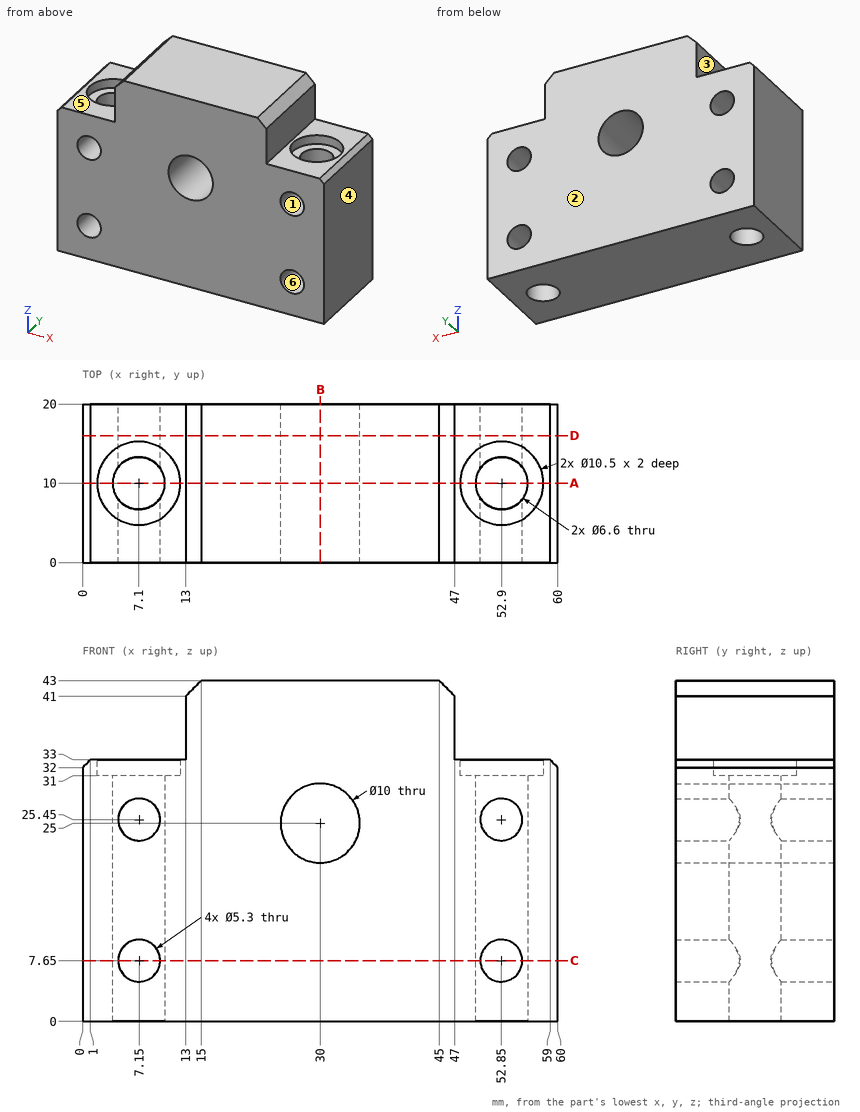
Drawing for the job (mm, zero at the part's lowest x, y, z). A direction names the side the tool comes from. Coordinates: 2 decimals unless noted, no trailing zeros. Order: outer loops, then holes, each group sorted by start corner. A loop starts at its lowest first (then second) coordinate and runs counter-clockwise, first axis right, second up.
Item 1: Band-saw the part on C-C on z = 7.65. List the corners of the cut face in (x, y), plus the area to 3 significant figures.
Check sheet entries:
outline: (0, 0) - (4.5, 0) - (4.5, 7.97) arc R3.3 cw to (4.5, 12.03) - (4.5, 20) - (0, 20) - close; (9.8, 0) - (50.2, 0) - (50.2, 8.1) arc R3.3 cw to (50.2, 11.9) - (50.2, 20) - (9.8, 20) - (9.8, 11.9) arc R3.3 cw to (9.8, 8.1) - close; (55.5, 0) - (60, 0) - (60, 20) - (55.5, 20) - (55.5, 12.03) arc R3.3 cw to (55.5, 7.97) - close
area: 981 mm2
Item 2: Band-saw the part on D-D on y = 16. List the corners of the cut face in (x, z).
Check sheet entries:
outline: (0, 0) - (60, 0) - (60, 32) - (59, 33) - (47, 33) - (47, 41) - (45, 43) - (15, 43) - (13, 41) - (13, 33) - (1, 33) - (0, 32) - close; hole circle Ø5.3 at (7.15, 7.65); hole circle Ø5.3 at (7.15, 25.45); hole circle Ø10 at (30, 25); hole circle Ø5.3 at (52.85, 7.65); hole circle Ø5.3 at (52.85, 25.45)
Item 3: Band-saw the part on A-A on y = 10. Give the number of separate pieces and of enclosed holes in the cut face, plus the area to 3 significant figures.
Check sheet entries:
separate pieces: 3
enclosed holes: 1
area: 1,790 mm2
Item 4: Two-plate mould, pull along X, no slides. Class the marked faces 1, 2, 3 and 4: +X half, -X half, draft (parallel to the pull), parting line (faces both ways), or undercut.
Check sheet entries:
face 1: undercut
face 2: draft
face 3: -X half
face 4: +X half
Item 5: Drill centre lines: L1, parallel to Z at x = 52.85, y = 13.75; L2, parallel to Z at x = 52.85, y = 17.75; L3, parallel to X at y = 4.25, z = 7.5. Where is each one in solid material? Low to high.
Check sheet entries:
L1: z = 0 to 5, 10.3 to 22.8, 28.1 to 31
L2: z = 0 to 5, 10.3 to 22.8, 28.1 to 33
L3: x = 0 to 4.5, 9.8 to 50.2, 55.5 to 60
Item 6: Pin check, flat tips, straight feed: pin 1 Ø6.5 at (y, z) = (9, 36) entering from +X; pin 2 Ø3.5 at (x, y) = (53, 12) entering from +Z; pin 3 Ø11.5 at (x, y) = (5.5, 7.5) entering from +Z. Stop position of each tip, or through.
Check sheet entries:
pin 1: stops at x = 59.25
pin 2: stops at z = 31
pin 3: stops at z = 33
Item 7: Band-saw the part on B-B on x = 30. List the corners of the cut face in (y, z), plus the area to 3 significant figures.
Check sheet entries:
outline: (0, 0) - (20, 0) - (20, 20) - (0, 20) - close; (0, 30) - (20, 30) - (20, 43) - (0, 43) - close
area: 660 mm2
Item 8: 3-axis set-ups, long thin cutter, end or side, ignore diameter. For the marked faces 5 and 6: which of +Z, -Z, +X, -X, +Y, -Y reach the whole face in a straight line?
Check sheet entries:
face 5: +Z, -X, +Y, -Y
face 6: +Y, -Y
